Could you check a few things on this model? Use its own coordinates, in mm. A direction names the side the tool comes from. Round coordinates to 2 decimals unless told otherwise and drop trailing zeros. Order: outer loops, then holes, each group sorted by start corner. A loop starts at its lowest first (then second) coordinate and runs counter-clockwise, first axis right, second up. Notation, with made-up numbers: (-6, 8) - (20, 8) arc R17 ccw to (20, 27) - close; hole circle Ø3 at (-10.5, 62.25). An arc over 180 degrees is marked (long way). Use one line per item in the form item = value.
from build123d import *

# Parameters (mm, degrees)
SKETCH1_W           = 95
SKETCH1_H           = 75
BOSS_EXTRUDE1_DEPTH = 10
SKETCH2_W           = 8
SKETCH2_H           = 20
REVOLVE1_ANGLE      = 180
SKETCH3_W           = 16
SKETCH3_H           = 20
BOSS_EXTRUDE2_DEPTH = 10
SKETCH4_R           = 17.178882312
CUT_EXTRUDE1_DEPTH  = 71.089228844
SWEEP2_START        = -8
SWEEP2_DEPTH        = 16


# Read off the part's stored shape, not the designer's step: Sweep2
with BuildPart() as part:
    # Sketch1 → Boss-Extrude1 (new, symmetric)
    with BuildSketch(Plane(origin=(0, 0, 0), x_dir=(1, 0, 0), z_dir=(0, 1, 0))):
        Rectangle(SKETCH1_W, SKETCH1_H)
    extrude(amount=BOSS_EXTRUDE1_DEPTH, both=True)

    # Sketch2 → Revolve1 (revolve)
    with BuildSketch(Plane.XY.offset(37.5)):
        with Locations((-4, 20)):
            Rectangle(SKETCH2_W, SKETCH2_H)
    revolve(axis=Axis((0, 10, 37.5), (0, -1, 0)), revolution_arc=REVOLVE1_ANGLE)

    # Sketch3 → Boss-Extrude2 (add)
    with BuildSketch(Plane.XY.offset(37.5)):
        with Locations((0, 20)):
            Rectangle(SKETCH3_W, SKETCH3_H)
    extrude(amount=BOSS_EXTRUDE2_DEPTH)

    # Sketch4 → Cut-Extrude1 (cut, through all)
    with BuildSketch(Plane(origin=(0, 10, 0), x_dir=(1, 0, 0), z_dir=(0, 1, 0))):
        with Locations(Location((0, 0, 0), (0, 0, 270))):
            Circle(SKETCH4_R)
    extrude(amount=-CUT_EXTRUDE1_DEPTH, mode=Mode.SUBTRACT)

    # Sweep2 outline → Sweep2 (add)
    with BuildSketch(Plane.YZ.offset(SWEEP2_START)):
        with BuildLine():
            ThreePointArc((30, 45), (31.767766953, 49.267766953), (27.5, 47.5))
            Line((27.5, 47.5), (30, 47.5))
            Line((30, 47.5), (30, 45))
        make_face()
    extrude(amount=SWEEP2_DEPTH)


solid = part.part
Item 1: If we mould it in two halves opening along X, with no side actions, what happens to faces 1 (the face through (-1, 0, 37.5)), 2 (the face through (8, 21, 42)), 3 (the face through (-10.453, 0.14, -13.633)), 4 (the face through (-8, 21, 42))? For each: released by +X, released by -X, zero draft, split by the parting line, or undercut.
Found:
face_1 = zero draft
face_2 = released by +X
face_3 = undercut
face_4 = released by -X
Item 2: Imagine slicing it at D-D on x = 0. Please give me the cut outline in (y, z), plus the area to 3 significant figures.
Found:
outline = (-10, -37.5) - (10, -37.5) - (10, -17.18) - (-10, -17.18) - close; (-10, 17.18) - (10, 17.18) - (10, 29.5) - (30, 29.5) - (30, 45) arc R2.5 ccw (long way) to (27.5, 47.5) - (10, 47.5) - (10, 37.5) - (-10, 37.5) - close
area = 1,190 mm2
Item 3: For faces 5 (the face through (0, 30, 37)), 6 (the face through (0, 19, 47.5)), 7 (the face through (-1, 0, -37.5)), 8 (the face through (-0.176, 20.14, 29.502)), which set-ups out of +Z, -Z, +X, -X, +Y, -Y let a thin tool reach every point of the face, with its end or its side?
Found:
face_5 = -Z, +X, -X, +Y
face_6 = +Z, +X, -X, -Y
face_7 = -Z, +X, -X, +Y, -Y
face_8 = -Z, +Y
Item 4: Imagine slicing it at C-C on y = -3.5. Please give me the cut outline in (x, z), plus the area to 3 significant figures.
Found:
outline = (-47.5, -37.5) - (47.5, -37.5) - (47.5, 37.5) - (-47.5, 37.5) - close; hole circle Ø34.36 at (0, 0)
area = 6,200 mm2
Item 5: Imagine slicing it at A-A on z = 0. Please give me the cut outline in (x, y).
Found:
outline = (-47.5, -10) - (-17.18, -10) - (-17.18, 10) - (-47.5, 10) - close; (17.18, -10) - (47.5, -10) - (47.5, 10) - (17.18, 10) - close
Item 6: Will these pins go through, and if not, where does the flat tip stop? P1, Ø1, axis at x = 37, z = -15.5, coming from the +Y side; P2, Ø17, axis at x = -2, z = 38, coming from the +Y side; P3, Ø1, axis at x = -5, y = 7, coming from the +Z side.
Found:
P1 = 10
P2 = 32.29
P3 = 37.5
Item 7: I need wall thicknesses on L1, parallel to X at y = -1, z = 0; L2, parallel to X at y = 17.5, z = 44.5; L3, parallel to Z at x = 40, y = 2.5. Which ranges of each line are inside material? Lowest first, please.
Found:
L1 = -47.5 to -17.18, 17.18 to 47.5
L2 = -8 to 8
L3 = -37.5 to 37.5
Item 8: Imagine slicing it at B-B on x = -10.5. Please give me the cut outline in (y, z), plus the area to 3 significant figures.
Found:
outline = (-10, -37.5) - (10, -37.5) - (10, -13.6) - (-10, -13.6) - close; (-10, 13.6) - (10, 13.6) - (10, 37.5) - (-10, 37.5) - close
area = 956 mm2
